CAD build for the part. Positions are in the model's coordinates, mm. A direction names the side the tool comes from. Round coordinates to 2 decimals unless told otherwise and drop trailing zeros. Order: outer loops, then holes, each group sorted by start corner. A loop starts at its lowest first (then second) coordinate and runs counter-clockwise, first axis right, second up. Notation, with made-up numbers: (-4, 82.5) -> (14, 82.5) arc R17 ccw to (14, 102.5) -> close; hole circle Ø2 at (-31, 13.25). An arc over 180 degrees is marked (long way). Return JSON: item names as keys, results as strings. Group by question number.
Q1. Flat gauge pins, fed straight in: pin 1 (4 mm diameter, centred on x = 4.5, y = 33, fed in from -Z); pin 2 (2.5 mm diameter, centred on x = -56, y = 1.5, fed in from +Z); pin 3 (6 mm diameter, centred on x = -61, y = 20.5, fed in from -Z); pin 4 (5 mm diameter, centred on x = -38.47, z = -38.47, fed in from -Y). Where does each tip first touch, or does it go through?
Q2. Mould opens along Z. For faces 6 (the cylindrical face through (1.1, 19.72, -62.99)), 7 (the cylindrical face through (-68, 20, 0)), 8 (the cylindrical face through (39.616, 1.521, -35.695)) say: +Z half, -Z half, draft (parallel to the pull), parting line (faces both ways), or undercut.
Q3. Cut at A-A (z = 0). Write the cut outline in (x, y), then the cut area to 3 significant figures.
Q4. Cut at B-B (x = 0). Write the cut outline in (y, z).
Q5. Cut at C-C (y = 29). Write the cut outline in (x, z), then the cut area to 3 significant figures.
Q6. Cut at D-D (z = -13). Write the cut outline in (x, y), then the cut area to 3 significant figures.
Q7. Probe line 1 along Z through (x, y) = (60, 25); line 2 along X through (y, z) = (2.25, -15); line 3 along Y through (x, z) = (46.5, 24.5). List the from-to ranges inside material, lowest first.
Q8. Which spindle directions (+Z, -Z, +X, -X, +Y, -Y) get a long thin tool onto all of the face, cutting with end or side? Do faces 1 (the flat face through (-62, 20, 20)), 2 (the flat face through (-62, 20, -20)), 3 (the cylindrical face through (-39.368, 1.521, 41.328)), 4 (the cylindrical face through (68, 20, 0)), 5 (the cylindrical face through (65, 21, 0)). Say none if no direction does.
from build123d import *

# Parameters (mm, degrees)
SKETCH1_R               = 68
BOSS_EXTRUDE1_DEPTH     = 40
CUT_EXTRUDE1_START      = -40
CUT_EXTRUDE1_DEPTH      = 40
SHELL1_T                = -3
CUT_EXTRUDE2_DEPTH      = 101.960388272
CUT_EXTRUDE2_DEPTH_BACK = 101.960388272
SKETCH3_R               = 3
SKETCH3_R_2             = 7.5
SKETCH4_R               = 3
CUT_EXTRUDE3_DEPTH      = 3
SKETCH6_W               = 15
SKETCH6_H               = 16
SKETCH6_W_2             = 11
SKETCH6_H_2             = 12
BOSS_EXTRUDE2_DEPTH     = 15
SKETCH7_W               = 4
SKETCH7_H               = 2.5
CUT_EXTRUDE5_DEPTH      = 3


with BuildPart() as part:
    # Sketch1 → Boss-Extrude1 (new body)
    with BuildSketch(Plane(origin=(0, 0, 0), x_dir=(1, 0, 0), z_dir=(0, 1, 0))):
        with Locations(Location((0, 0, 0), (0, 0, 270))):
            Circle(SKETCH1_R)
    extrude(amount=BOSS_EXTRUDE1_DEPTH)

    # Sketch2 → Cut-Extrude1 (cut)
    with BuildSketch(Plane(origin=(0, 40, 0), x_dir=(1, 0, 0), z_dir=(0, 1, 0)).offset(CUT_EXTRUDE1_START)):
        with BuildLine():
            Line((-59.741108125, -20), (-64.992307237, -20))
            ThreePointArc((-64.992307237, -20), (0, -68), (64.992307237, -20))
            Line((64.992307237, -20), (59.741108125, -20))
            ThreePointArc((59.741108125, -20), (0, -63), (-59.741108125, -20))
        make_face()
        with BuildLine():
            Line((-59.741108125, 20), (-64.992307237, 20))
            ThreePointArc((-64.992307237, 20), (0, 68), (64.992307237, 20))
            Line((64.992307237, 20), (59.741108125, 20))
            ThreePointArc((59.741108125, 20), (0, 63), (-59.741108125, 20))
        make_face()
    extrude(amount=CUT_EXTRUDE1_DEPTH, mode=Mode.SUBTRACT)

    # Shell1
    shell1_openings = [part.faces().sort_by_distance(p)[0] for p in [
        (0, 40, 0),
    ]]
    offset(amount=SHELL1_T, openings=shell1_openings, kind=Kind.INTERSECTION)

    # Sketch3 → Cut-Extrude2 (cut, two sides: drawn at the far end of the back side and taken through both)
    with BuildSketch(Plane.XZ.offset(-CUT_EXTRUDE2_DEPTH_BACK)):
        with Locations(Location((-38.466608897, 38.466608897, 0), (0, 0, 90))):
            Circle(SKETCH3_R)
        with Locations(Location((38.466608897, -38.466608897, 0), (0, 0, 90))):
            Circle(SKETCH3_R)
        with Locations(Location((0, 30, 0), (0, 0, 90))):
            Circle(SKETCH3_R_2)
        with Locations(Location((25.980762114, 15, 0), (0, 0, 90))):
            Circle(SKETCH3_R_2)
        with Locations(Location((25.980762114, -15, 0), (0, 0, 90))):
            Circle(SKETCH3_R_2)
        with Locations(Location((0, -30, 0), (0, 0, 90))):
            Circle(SKETCH3_R_2)
        with Locations(Location((-25.980762114, -15, 0), (0, 0, 90))):
            Circle(SKETCH3_R_2)
        with Locations(Location((-25.980762114, 15, 0), (0, 0, 90))):
            Circle(SKETCH3_R_2)
        with Locations(Location((-38.466608897, -38.466608897, 0), (0, 0, 90))):
            Circle(SKETCH3_R)
        with Locations(Location((38.466608897, 38.466608897, 0), (0, 0, 90))):
            Circle(SKETCH3_R)
    extrude(amount=CUT_EXTRUDE2_DEPTH + CUT_EXTRUDE2_DEPTH_BACK, mode=Mode.SUBTRACT)

    # Sketch4 → Cut-Extrude3 (cut)
    with BuildSketch(Plane(origin=(0, 3, 0), x_dir=(1, 0, 0), z_dir=(0, 1, 0))):
        with Locations(Location((0, 0, 0), (0, 0, 270))):
            Circle(SKETCH4_R)
    extrude(amount=-CUT_EXTRUDE3_DEPTH, mode=Mode.SUBTRACT)

    # Sketch6 → Boss-Extrude2 (add)
    with BuildSketch(Plane(origin=(0, 3, 0), x_dir=(1, 0, 0), z_dir=(0, 1, 0))):
        with Locations((-55.5, 0)):
            Rectangle(SKETCH6_W, SKETCH6_H)
        with Locations((-55.5, 0)):
            Rectangle(SKETCH6_W_2, SKETCH6_H_2, mode=Mode.SUBTRACT)
    extrude(amount=BOSS_EXTRUDE2_DEPTH)

    # Sketch7 → Cut-Extrude5 (cut)
    with BuildSketch(Plane(origin=(0, 3, 0), x_dir=(1, 0, 0), z_dir=(0, 1, 0))):
        with Locations((-55.5, -4.75)):
            Rectangle(SKETCH7_W, SKETCH7_H)
    extrude(amount=-CUT_EXTRUDE5_DEPTH, mode=Mode.SUBTRACT)


solid = part.part
Solution:
{
 "1": {"pin 1": "stops at z = -62.95", "pin 2": "stops at z = 31.17", "pin 3": "stops at z = -24.6", "pin 4": "passes through"},
 "2": {"face 6": "-Z half", "face 7": "parting line", "face 8": "undercut"},
 "3": {"outline": "(-68, 0) -> (-3, 0) -> (-3, 3) -> (-48, 3) -> (-48, 18) -> (-50, 18) -> (-50, 3) -> (-61, 3) -> (-61, 18) -> (-63, 18) -> (-63, 3) -> (-65, 3) -> (-65, 40) -> (-68, 40) -> close; (3, 0) -> (68, 0) -> (68, 40) -> (65, 40) -> (65, 3) -> (3, 3) -> close", "area": "672 mm²"},
 "4": {"outline": "(0, -63) -> (40, -63) -> (40, -60) -> (3, -60) -> (3, -37.5) -> (0, -37.5) -> close; (0, -22.5) -> (3, -22.5) -> (3, -3) -> (0, -3) -> close; (0, 3) -> (3, 3) -> (3, 22.5) -> (0, 22.5) -> close; (0, 37.5) -> (3, 37.5) -> (3, 60) -> (40, 60) -> (40, 63) -> (0, 63) -> close"},
 "5": {"outline": "(-64.99, -20) -> (-59.74, -20) arc R63 ccw to (59.74, -20) -> (64.99, -20) arc R68 ccw to (64.99, 20) -> (59.74, 20) arc R63 ccw to (-59.74, 20) -> (-64.99, 20) arc R68 ccw to start; hole (-62.74, -17) -> (-57.54, -17) arc R60 ccw to (57.54, -17) -> (62.74, -17) arc R65 ccw to (62.74, 17) -> (57.54, 17) arc R60 ccw to (-57.54, 17) -> (-62.74, 17) arc R65 ccw to start", "area": "1,220 mm²"},
 "6": {"outline": "(-66.75, 0) -> (-33.21, 0) -> (-33.21, 3) -> (-63.69, 3) -> (-63.69, 40) -> (-66.75, 40) -> close; (-18.75, 0) -> (18.75, 0) -> (18.75, 3) -> (-18.75, 3) -> close; (33.21, 0) -> (66.75, 0) -> (66.75, 40) -> (63.69, 40) -> (63.69, 3) -> (33.21, 3) -> close", "area": "540 mm²"},
 "7": {"line 1": "z = -20 to -17, 17 to 20", "line 2": "x = -66.32 to -33.48, -18.48 to 18.48, 33.48 to 66.32", "line 3": "y = 0 to 3"},
 "8": {"face 1": "+Z, -X, +Y, -Y", "face 2": "-Z, -X, +Y, -Y", "face 3": "+Y, -Y", "face 4": "+X, +Y, -Y", "face 5": "+Y"}
}
